Could you check a few things on this model? Use its own coordinates, in mm. Give positions to 0.01 mm unless a question says otherwise; leave off trailing zeros. Write each loop counter-clockwise with the first axis right and the second up, starting at its lowest first coordinate (ties: lowest second). Pieces come first, ordered by that corner, then holes. Notation, with made-up numbers: (65.25, 50.25) - (113.25, 50.25) arc R25 ccw to (113.25, 69.25) - close; hole circle Ø8 at (-31.75, 50.5). An arc over 180 degrees is marked (long way). Answer in a Markdown table with one row per item.
from build123d import *

# Parameters (mm, degrees)
SKETCH_1_W                  = 6
SKETCH_1_H                  = 30
EXTRUDE_1_DEPTH             = 247
SKETCH_2_R                  = 22.5
EXTRUDE_2_DEPTH             = 6
SKETCH_3_R                  = 13
CUT_EXTRUDE_1_DEPTH         = 250.90248098
HOLE_WIZARD_M31_D           = 3.4
HOLE_WIZARD_M31_CBORE_D     = 6.7
HOLE_WIZARD_M31_CBORE_DEPTH = 2
HOLE_WIZARD_M41_D           = 4.5
EXTRUDE_3_DEPTH             = 6
M3X0_51_D                   = 2.5
M3X0_51_DEPTH               = 8.5
M3X0_51_TIP                 = 0.751075774
M3X0_52_D                   = 2.5
M3X0_52_DEPTH               = 8.5
M3X0_52_TIP                 = 0.751075774


with BuildPart() as part:
    # Эскиз1 → Бобышка-Вытянуть1 (new body)
    with BuildSketch(Plane(origin=(0, 0, 0), x_dir=(1, 0, 0), z_dir=(0, 1, 0))):
        with Locations((3, -15)):
            Rectangle(SKETCH_1_W, SKETCH_1_H)
    extrude(amount=EXTRUDE_1_DEPTH)

    # Эскиз2 → Бобышка-Вытянуть2 (add)
    with BuildSketch(Plane.ZY):
        with Locations((15, 123.5)):
            Circle(SKETCH_2_R)
    extrude(amount=-EXTRUDE_2_DEPTH)

    # Эскиз3 → Вырез-Вытянуть1 (cut, through all)
    with BuildSketch(Plane.ZY):
        with Locations((15, 123.5)):
            Circle(SKETCH_3_R)
    extrude(amount=-CUT_EXTRUDE_1_DEPTH, mode=Mode.SUBTRACT)

    # Цековка для  винта с полукруглой головкой M31 (through all)
    with Locations(Plane(origin=(6, -25.024735225, 7.262908886), x_dir=(0, 0, 1), z_dir=(1, 0, 0))):
        with Locations((7.737091114, -167.774735225), (-11.512908886, -148.524735225), (7.737091114, -129.274735225), (26.987091114, -148.524735225)):
            CounterBoreHole(HOLE_WIZARD_M31_D / 2, HOLE_WIZARD_M31_CBORE_D / 2, HOLE_WIZARD_M31_CBORE_DEPTH)

    # Отверстие с зазором M41 (through all)
    with Locations(Plane(origin=(6, 0, 0), x_dir=(0, 0, -1), z_dir=(1, 0, 0))):
        with Locations((-26, 163.5), (-4, 163.5), (-4, 83.5), (-26, 83.5)):
            Hole(HOLE_WIZARD_M41_D / 2)

    # Эскиз11 → Бобышка-Вытянуть3 (add)
    with BuildSketch(Plane(origin=(6, 0, 0), x_dir=(0, 0, -1), z_dir=(1, 0, 0))):
        Polygon((-37.5, 241), (-30, 228.009618943), (0, 228.009618943), (7.5, 241), (7.5, 247), (-37.5, 247), align=None)
        Polygon((0, 18.990381057), (7.5, 6), (7.5, 0), (-37.5, 0), (-37.5, 6), (-30, 18.990381057), align=None)
    extrude(amount=-EXTRUDE_3_DEPTH)

    # Отверстие обработанное метчиком M3x0.51
    with Locations(Plane(origin=(0, 0, 0), x_dir=(-1, 0, 0), z_dir=(0, -1, 0))):
        with Locations((-3, -28.5), (-3, -19.5), (-3, -10.5), (-3, -1.5)):
            Hole(M3X0_51_D / 2, depth=M3X0_51_DEPTH)
            with Locations((0, 0, -(M3X0_51_DEPTH + M3X0_51_TIP / 2))):  # 118° drill point
                Cone(0, M3X0_51_D / 2, M3X0_51_TIP, mode=Mode.SUBTRACT)

    # Отверстие обработанное метчиком M3x0.52
    with Locations(Plane(origin=(0, 247, 0), x_dir=(1, 0, 0), z_dir=(0, 1, 0))):
        with Locations((3, -1.5), (3, -10.5), (3, -19.5), (3, -28.5)):
            Hole(M3X0_52_D / 2, depth=M3X0_52_DEPTH)
            with Locations((0, 0, -(M3X0_52_DEPTH + M3X0_52_TIP / 2))):  # 118° drill point
                Cone(0, M3X0_52_D / 2, M3X0_52_TIP, mode=Mode.SUBTRACT)


solid = part.part
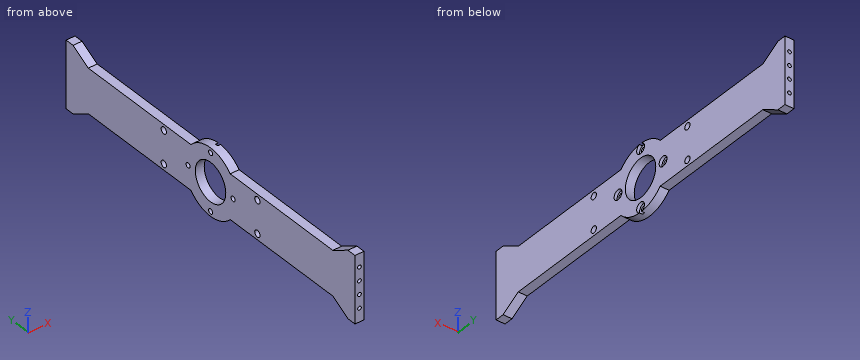
1) Imagine slicing it at A-A (y = 83.5). List the corners of the cut face in (x, z) for me.
Check values:
| item | result |
|---|---|
| outline | (0, 0) - (6, 0) - (6, 1.75) - (0, 1.75) - close; (0, 6.25) - (6, 6.25) - (6, 23.75) - (0, 23.75) - close; (0, 28.25) - (6, 28.25) - (6, 30) - (0, 30) - close |
2) Will these pins go through, and if not, where does the flat tip stop? P1, Ø2, axis at x = 3, z = 10.5, coming from the +Y side; P2, Ø3.5, axis at y = 142, z = 15.5, coming from the +X side; P3, Ø2, axis at x = 3, z = 19.5, coming from the -Y side.
Check values:
| item | result |
|---|---|
| P1 | stops at y = 238.35 |
| P2 | stops at x = 4 |
| P3 | stops at y = 8.65 |
3) Imagine slicing it at B-B (y = 35.5). List the corners of the cut face in (x, z) for me.
Check values:
| item | result |
|---|---|
| outline | (0, 0) - (6, 0) - (6, 30) - (0, 30) - close |
4) If I drill on line 1 (X direction, y = 4.25, z = 28.5); line 2 (Y direction, x = 4.8, z = 13); line 3 (Y direction, x = 3.55, z = -4.5), over which ranges is the centre line in solid material (lowest first)?
Check values:
| item | result |
|---|---|
| line 1 | x = 0 to 1.75, 4.25 to 6 |
| line 2 | y = 0 to 101.56, 106.94 to 110.65, 136.35 to 140.06, 145.44 to 247 |
| line 3 | y = 0 to 11.2, 112.28 to 121.82, 125.18 to 134.72, 235.8 to 247 |
